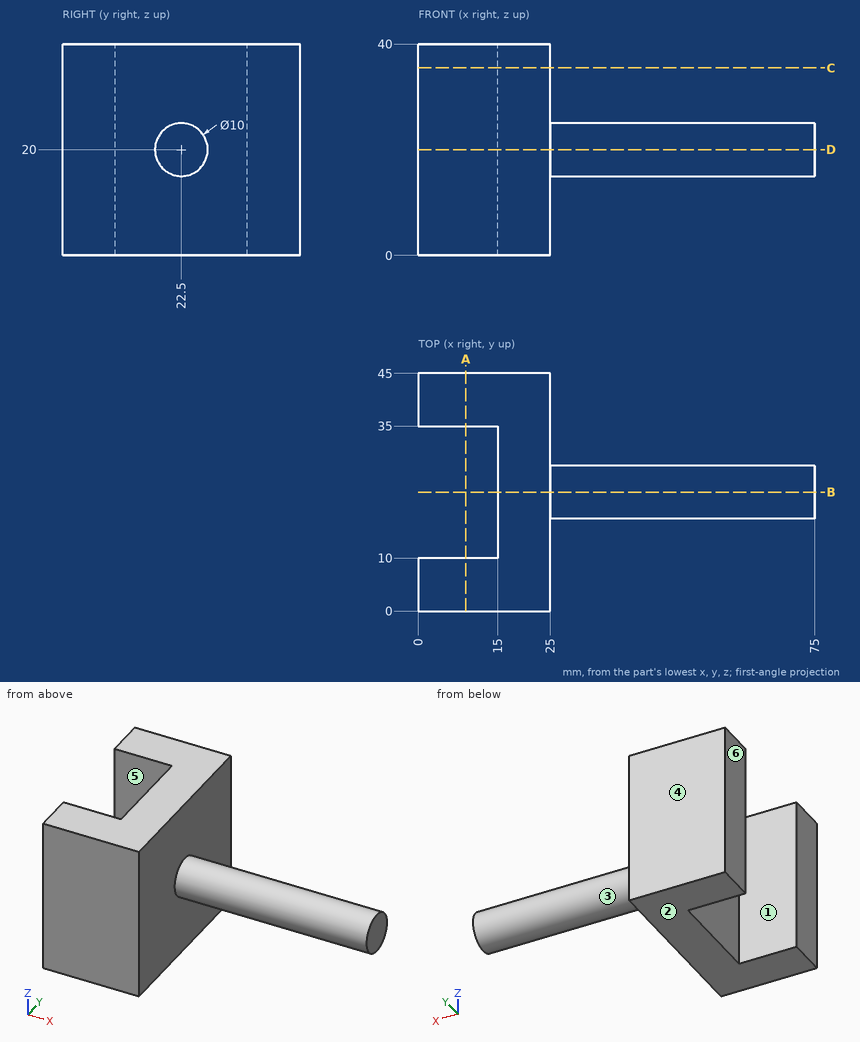
Check sheet for the drawn part. Datum: minimum x, y, z corner. Units: mm. A direction names the side the tool comes from. Give positions to 0.01 mm unless a question says otherwise; leave off trailing zeros. Loops run counter-clockwise (first coordinate to the right, second up) from the corner with the lowest first, then second, coordinate; pieces in that order, holes last. Notation, with made-up numbers: M 46.25,-30 L 51.25,-30 A16 cw 51.25,-16 Z; hole C 83,-14.5 d4. An arc over 180 degrees is marked long. Answer as CSV lines item,"result".
Item 1: Sectioned sample at B-B, the plane y = 22.5. Enter the section's corners in (x, z).
Reply:
outline,"M 15,0 L 25,0 L 25,15 L 75,15 L 75,25 L 25,25 L 25,40 L 15,40 Z"
Item 2: Sectioned sample at A-A, the plane x = 9. Enter the section's corners in (y, z).
Reply:
outline,"M 0,0 L 10,0 L 10,40 L 0,40 Z; M 35,0 L 45,0 L 45,40 L 35,40 Z"
Item 3: Depth check by flat-ended pin: pin 1 Ø4 at (y, z) = (31, 34) entering from -X; pin 2 Ø2 at (y, z) = (33.5, 8) entering from +X; pin 3 Ø6 at (x, y) = (55.5, 21) entering from -Z. Enter the tip coordinate at first touch or a pass-through.
Reply:
pin 1,"x = 15"
pin 2,"x = 25"
pin 3,"z = 15"
Item 4: Set-up check for the marked faces 1 and 2: record each of +Z, -Z, +X, -X, +Y, -Y from which the full face is reachable in a straight line by a thin tool's end or side.
Reply:
face 1,"+Z, -Z, -X"
face 2,"-Z, +X, -X, +Y, -Y"
Item 5: Draft check along Y on the marked faces 3, 4, 5 and 6. Enter one of: pulls with the +Y half, pulls with the -Y half, needs draft (parallel to the pull), parting line crosses it, or undercut.
Reply:
face 3,"parting line crosses it"
face 4,"pulls with the +Y half"
face 5,"undercut"
face 6,"needs draft"
Item 6: Sectioned sample at C-C, the plane z = 35.5. Enter the section's corners in (x, y), then the cut area to 3 significant figures.
Reply:
outline,"M 0,0 L 25,0 L 25,45 L 0,45 L 0,35 L 15,35 L 15,10 L 0,10 Z"
area,"750 mm^2"
Item 7: Sectioned sample at D-D, the plane z = 20. Enter the section's corners in (x, y), then the cut area to 3 significant figures.
Reply:
outline,"M 0,0 L 25,0 L 25,17.5 L 75,17.5 L 75,27.5 L 25,27.5 L 25,45 L 0,45 L 0,35 L 15,35 L 15,10 L 0,10 Z"
area,"1,250 mm^2"
Item 8: Scan lines: L1, parallel to Y at x = 13.5, z = 25.5; L2, parallel to X at y = 14, z = 24; L3, parallel to X at y = 35.5, z = 30.5. Record each from-to range of solid material in increasing order.
Reply:
L1,"0 to 10, 35 to 45"
L2,"15 to 25"
L3,"0 to 25"
